Autodesk Inventor part; units mm, degrees
ref_plane "YZ Plane" through (0, 0, 0) normal (1, 0, 0) x (0, 1, 0)
ref_plane "XZ Plane" through (0, 0, 0) normal (0, 1, 0) x (-1, 0, 0)
ref_plane "XY Plane" through (0, 0, 0) normal (0, 0, 1) x (1, 0, 0)
sketch "Эскиз1" plane through (0, 0, 0) normal (1, 0, 0) x (0, 1, 0)
  line L0 (-7, 7) -> (7, 7)
  line L1 (7, 7) -> (7, -7)
  line L2 (7, -7) -> (-7, -7)
  line L3 (-7, -7) -> (-7, 7)
  line L4 (-7, 7) -> (7, -7) construction
  line L5 (7, 7) -> (-7, -7) construction
  line L6 (0, 9) -> (0, -9)
  circle A0 centre (0, -9) radius 2
  circle A1 centre (0, 9) radius 2
  line L7 (2, 9) -> (2, -9)
  line L8 (-2, -9) -> (-2, 9)
  line L9 (4.25, 4.25) -> (-4.25, 4.25)
  line L10 (-4.25, 4.25) -> (-4.25, -4.25)
  line L11 (-4.25, -4.25) -> (4.25, -4.25)
  line L12 (4.25, -4.25) -> (4.25, 4.25)
  line L13 (4.25, 4.25) -> (-4.25, -4.25) construction
  line L14 (-4.25, 4.25) -> (4.25, -4.25) construction
  line L15 (-7, 4) -> (-11, 4)
  line L16 (-11, 4) -> (-11, -4)
  line L17 (-11, -4) -> (-7, -4)
  line L18 (-7, -4) -> (-7, 4)
  circle A2 centre (0, 9) radius 1
  circle A3 centre (0, -9) radius 1
  line L19 (-7, 0) -> (-11, 0)
  line L20 (-7, 4) -> (-4.25, 4)
  line L21 (-4.25, 4) -> (-4.25, -4)
  line L22 (-4.25, -4) -> (-7, -4)
  line L23 (-7, -4) -> (-7, 4)
  point P0 (0, 0)
  point P1 (0, 0)
  point P2 (2, -7)
  point P3 (2, 7)
  point P4 (-2, 7)
  point P5 (-7, -4)
  point P6 (-2, -7)
  point P7 (-7, 0)
  dimension "d0" = 14
  dimension "d1" = 14
  dimension "d2" = 18
  dimension "d3" = 8.5
  dimension "d4" = 8.5
  dimension "d5" = 4
  dimension "d6" = 2
  dimension "d7" = 2
  dimension "d14" = 8
extrude "Выдавливание1" add sketch "Эскиз1" along normal blind 0.2 contours L20 L10 L22 L3 | L3 L19 L16 L15 | L9 L6 L11 L8 | L8 L11 L10 L9 | L3 L17 L16 L19 | L9 L7 L11 L6 | L9 L12 L11 L7
sketch "Эскиз2" plane through (0, 0, 0) normal (-1, 0, 0) x (0, 0, 1)
  line L0 (-4.25, 4.25) -> (4.25, 4.25)
  line L1 (4.25, 4.25) -> (4.25, -4.25)
  line L2 (4.25, -4.25) -> (-4.25, -4.25)
  line L3 (-4.25, -4.25) -> (-4.25, 4.25)
  line L4 (-4.25, 4.25) -> (4.25, -4.25) construction
  line L5 (4.25, 4.25) -> (-4.25, -4.25) construction
  point P0 (0, 0)
  dimension "d10" = 8.5
  dimension "d11" = 8.5
extrude "Выдавливание2" add sketch "Эскиз2" against normal blind 5.3
properties part number "imx258"
Input: part model. Units: mm. Frame: model coordinates. A direction names the side the tool comes from. Round coordinates to 2 decimals unless told otherwise and drop trailing zeros. Write each loop counter-clockwise with the first axis right and the second up, starting at its lowest first coordinate (ties: lowest second). Pieces come first, ordered by that corner, then holes.
1) Cut plane A-A (z = 3). Return the cut outline in (x, y), then the cut area to 3 significant figures.
2) Ray query, L1, parallel to Y at x = 4.85, z = 3.75; L2, parallel to X at y = -9.75, z = 0.75. Return the intervals inside material, ascending.
3) Contact query for flat-ended pins moving along their axis: P1, Ø1, axis at y = -3.5, z = -1, coming from the -X side; P2, Ø3, axis at x = 2.5, y = -8.5, coming from the +Z side; P3, Ø2.5, axis at x = 2, z = -1, coming from the -Y side; P4, Ø1.5, axis at y = -5.5, z = 0.5, coming from the +X side. Output: stop coordinate, or through.
4) Reachability of faces 1 (the flat face through (0.2, -8, 0)), 2 (the flat face through (3, 0, 4.25)) from +Z, -Z, +X, -X, +Y, -Y: full face, straight path, thin tool, end or side. Return the list, or none.
5) Cut plane C-C (x = 0.6). Return the cut outline in (y, z), then the cut area to 4 significant figures.
6) Cut plane B-B (y = -5). Return the cut outline in (x, z).
Geometry says:
1. outline: (0, -11) - (0.2, -11) - (0.2, -4.25) - (5.3, -4.25) - (5.3, 4.25) - (0, 4.25) - close
1. area: 46.4 mm2
2. L1: y = -4.25 to 4.25
2. L2: x = 0 to 0.2
3. P1: stops at x = 0
3. P2: passes through
3. P3: stops at y = -4.25
3. P4: stops at x = 0.2
4. face 1: +Z, -Z, +X, -Y
4. face 2: +Z, +X, -X, +Y, -Y
5. outline: (-4.25, -4.25) - (4.25, -4.25) - (4.25, 4.25) - (-4.25, 4.25) - close
5. area: 72.25 mm2
6. outline: (0, -4) - (0.2, -4) - (0.2, 4) - (0, 4) - close
